```python
from build123d import *

# Parameters (mm, degrees)
BOSS_EXTRUDE1_DEPTH = 300


with BuildPart() as part:
    # Sketch2 → Boss-Extrude1 (new body, symmetric)
    with BuildSketch(Plane.XY):
        with BuildLine():
            Line((-50, 40), (-50, -40))
            ThreePointArc((-50, -40), (-47.071067812, -47.071067812), (-40, -50))
            Line((-40, -50), (40, -50))
            ThreePointArc((40, -50), (47.071067812, -47.071067812), (50, -40))
            Line((50, -40), (50, 40))
            ThreePointArc((50, 40), (47.071067812, 47.071067812), (40, 50))
            Line((40, 50), (-40, 50))
            ThreePointArc((-40, 50), (-47.071067812, 47.071067812), (-50, 40))
        make_face()
        with BuildLine():
            Line((40, 45), (-40, 45))
            ThreePointArc((-40, 45), (-43.535533906, 43.535533906), (-45, 40))
            Line((-45, 40), (-45, -40))
            ThreePointArc((-45, -40), (-43.535533906, -43.535533906), (-40, -45))
            Line((-40, -45), (40, -45))
            ThreePointArc((40, -45), (43.535533906, -43.535533906), (45, -40))
            Line((45, -40), (45, 40))
            ThreePointArc((45, 40), (43.535533906, 43.535533906), (40, 45))
        make_face(mode=Mode.SUBTRACT)
    extrude(amount=BOSS_EXTRUDE1_DEPTH, both=True)


solid = part.part
```
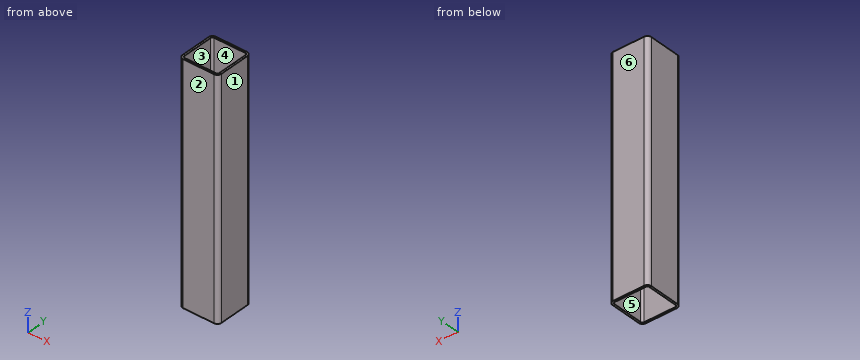
CAD build for the part. Positions are in the model's coordinates, mm. Face numbers are marked on the shaded views. A direction names the side the tool comes from. Give positions to 0.01 mm unless a question says otherwise; leave off trailing zeros. Loops run counter-clockwise (first coordinate to the right, second up) from the corner with the lowest first, then second, coordinate; pieces in that order, holes last. Notation, with made-up numbers: (-6, 12.25) -> (40, 12.25) arc R9 ccw to (40, 22.25) -> close; hole circle Ø3 at (47, -14.75). An arc over 180 degrees is marked (long way). Use a Markdown table: item, result.
1. Mould opens along X. For the marked faces 1, 2, 3 and 4 say: pulls with the +X half, pulls with the -X half, needs draft (parallel to the pull), parting line crosses it, or undercut.
Check result:
| item | result |
|---|---|
| face 1 | pulls with the +X half |
| face 2 | needs draft |
| face 3 | undercut |
| face 4 | undercut |
2. Which spindle directions (+Z, -Z, +X, -X, +Y, -Y) get a long thin tool onto all of the face, cutting with end or side? Do the marked faces 5 and 6. Say none if no direction does.
Check result:
| item | result |
|---|---|
| face 5 | +Z, -Z |
| face 6 | +Z, -Z, +X, -X, +Y |
3. Wall check: L1, parallel to X at y = -1, z = 161; L2, parallel to Y at x = -40.5, z = 75; L3, parallel to X at y = -43, z = 26. Give the ranges that are in metal, low to high. Write a range as [from, to].
Check result:
| item | result |
|---|---|
| L1 | x = [-50, -45], [45, 50] |
| L2 | y = [-49.99, -44.97], [44.97, 49.99] |
| L3 | x = [-49.54, -44], [44, 49.54] |
4. Slice it at A-A (x = -33.5). List the corners of the cut face in (y, z).
Check result:
| item | result |
|---|---|
| outline | (-50, -300) -> (-45, -300) -> (-45, 300) -> (-50, 300) -> close; (45, -300) -> (50, -300) -> (50, 300) -> (45, 300) -> close |
5. Slice it at C-C (z = 148.5). List the corners of the cut face in (x, y).
Check result:
| item | result |
|---|---|
| outline | (-50, -40) arc R10 ccw to (-40, -50) -> (40, -50) arc R10 ccw to (50, -40) -> (50, 40) arc R10 ccw to (40, 50) -> (-40, 50) arc R10 ccw to (-50, 40) -> close; hole (-45, -40) arc R5 ccw to (-40, -45) -> (40, -45) arc R5 ccw to (45, -40) -> (45, 40) arc R5 ccw to (40, 45) -> (-40, 45) arc R5 ccw to (-45, 40) -> close |
